For this review, take the finished solid that the model builds, in its own axes (mm). Coordinates: 2 decimals unless noted, no trailing zeros. Write each loop counter-clockwise with the first axis right and the second up, starting at its lowest first coordinate (ties: lowest second). Pieces come first, ordered by that corner, then holes. Notation, with made-up numbers: M -34,37 L 11,37 A20 ccw 11,65 Z; hole C 62,35.5 d8. An arc over 180 degrees is marked long. One line per question, with ' | ' between items.
from build123d import *

# Parameters (mm, degrees)
F0_W           = 44.45
F0_H           = 44.45
F1_DEPTH       = 544.5125
F3_D           = 20.6375
F3_CSINK_D     = 38.1
F3_CSINK_ANGLE = 82


with BuildPart() as f1:
    # F0 (on Right) → F1 (new body, symmetric)
    with BuildSketch(Plane.YZ):
        with Locations((0, 22.225)):
            Rectangle(F0_W, F0_H)
    extrude(amount=F1_DEPTH, both=True)

    # F3 (through all)
    with Locations(Plane.XY.offset(44.45)):
        with Locations((-508, 0), (-254, 0), (0, 0), (254, 0), (508, 0)):
            CounterSinkHole(F3_D / 2, F3_CSINK_D / 2, counter_sink_angle=F3_CSINK_ANGLE)


solid = f1.part
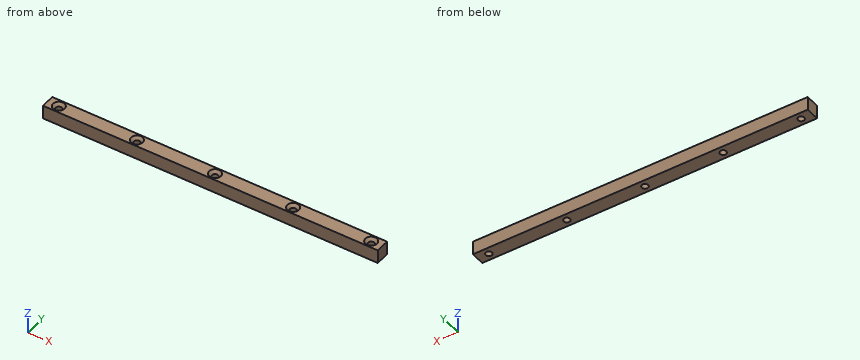
1. Take a section at C-C on z = 26. State the section outline as (x, y) points (1 decimal), plus the area to 3 significant figures.
Computed values:
outline: M -544.5,-22.2 L 544.5,-22.2 L 544.5,22.2 L -544.5,22.2 Z; hole C -508,0 d20.6; hole C -254,0 d20.6; hole C 0,0 d20.6; hole C 254,0 d20.6; hole C 508,0 d20.6 | area: 46,700 mm2
2. For line 1 along X through (y, z) = (0, 8); line 2 along Y through (x, z) = (-254, 13.5) (3 decimals); line 3 along X through (y, z) = (-6, 18.5), list the stretches that pass through material, from the lowest coordinate up.
Computed values:
line 1: x = -544.51 to -518.32, -497.68 to -264.32, -243.68 to -10.32, 10.32 to 243.68, 264.32 to 497.68, 518.32 to 544.51 | line 2: y = -22.225 to -10.319, 10.319 to 22.225 | line 3: x = -544.51 to -516.4, -499.6 to -262.4, -245.6 to -8.4, 8.4 to 245.6, 262.4 to 499.6, 516.4 to 544.51
3. Take a section at B-B on x = -508. State the section outline as (y, z) points (3 decimals), plus the area to 3 significant figures.
Computed values:
outline: M -22.225,0 L -10.319,0 L -10.319,34.406 L -19.05,44.45 L -22.225,44.45 Z; M 10.319,0 L 22.225,0 L 22.225,44.45 L 19.05,44.45 L 10.319,34.406 Z | area: 971 mm2
4. Take a section at A-A on y = 0. Give the number of separate pieces and of enclosed holes in the cut face, plus the area to 3 significant figures.
Computed values:
separate pieces: 6 | enclosed holes: 0 | area: 43,400 mm2
